Design review of the part built by this model. Coordinates are the model's own, in mm. A direction names the side the tool comes from. Coordinates: 2 decimals unless noted, no trailing zeros. Loops run counter-clockwise (first coordinate to the right, second up) from the corner with the lowest first, then second, coordinate; pieces in that order, holes last. Notation, with made-up numbers: (81, 70.25) -> (102, 70.25) arc R23 ccw to (102, 93.25) -> close; hole circle Ø5 at (57.25, 55.5). An arc over 180 degrees is marked (long way). Use one line per item in the form item = value. Start each with the question number.
1. Wall thickness on line 1 (Y direction, x = 249, z = 26.5); line 2 (Y direction, x = 162, z = -16); line 3 (Z direction, x = 71, y = 4.5): over which ranges is each line inside the solid? List them lowest first. Write a range as from..to.
2. The part is to be moulded in two halves that separate along Y. For faces 5 (the face through (119.259, -30.742, 30.07)), 6 (the face through (120.595, 37.245, 29.93)), 7 (the face through (118, 7, 71)), say which applies: released by +Y, released by -Y, zero draft, split by the parting line, or undercut.
3. For pin 1 (5 mm diameter, centred on x = 209, z = 30, fed in from -Y); pin 2 (6 mm diameter, centred on y = 25.5, z = 31, fed in from +X); pin 3 (5 mm diameter, centred on y = 1.5, z = 3, fed in from +X), all flat-tipped, find the tip position at first contact; note any pin that passes through.
4. Consider section B-B (y = 20.5). State the section outline as (x, z) points, then the cut area to 3 significant figures.
5. Consider section C-C (z = 21.5). State the section outline as (x, y) points, then the cut area to 3 significant figures.
6. Machinability: for faces 1 (the face through (119.281, -29.742, 29.93)), 2 (the face through (251, 7, 31)), 3 (the face through (120, 38, 35)), 4 (the face through (-11, 7, 31)), which of the approach directions +Z, -Z, +X, -X, +Y, -Y give a long, thin tool a straight path to every point of the face, cutting with its end or side? Answer none if there is none.
7. Consider section D-D (y = -3). State the section outline as (x, z) points, then the cut area to 3 significant figures.
8. Consider section A-A (x = 120). State the section outline as (y, z) points, then the cut area to 4 significant figures.
from build123d import *

# Parameters (mm, degrees)
SKETCH1_W           = 262
SKETCH1_H           = 82
BOSS_EXTRUDE1_DEPTH = 10
SKETCH2_W           = 282
SKETCH2_H           = 102
BOSS_EXTRUDE2_DEPTH = 1.25
SKETCH3_R           = 34.5
SKETCH3_R_2         = 33.5
BOSS_EXTRUDE3_DEPTH = 5


with BuildPart() as part:
    # Sketch1 → Boss-Extrude1 (new body)
    with BuildSketch(Plane(origin=(0, 2.5, 0), x_dir=(1, 0, 0), z_dir=(0, 1, 0))):
        with Locations((120, -30)):
            Rectangle(SKETCH1_W, SKETCH1_H)
    extrude(amount=BOSS_EXTRUDE1_DEPTH)

    # Sketch2 → Boss-Extrude2 (add)
    with BuildSketch(Plane(origin=(0, 12.5, 0), x_dir=(1, 0, 0), z_dir=(0, 1, 0))):
        with Locations((120, -30)):
            Rectangle(SKETCH2_W, SKETCH2_H)
    extrude(amount=BOSS_EXTRUDE2_DEPTH)

    # Sketch3 → Boss-Extrude3 (add, symmetric)
    with BuildSketch(Plane.XY.offset(30)):
        with Locations((120, 3.75)):
            Circle(SKETCH3_R)
        with Locations((120, 3.75)):
            Circle(SKETCH3_R_2, mode=Mode.SUBTRACT)
    extrude(amount=BOSS_EXTRUDE3_DEPTH, both=True)


solid = part.part
Geometry check:
q1.line_1 = 2.5..13.75
q1.line_2 = 12.5..13.75
q1.line_3 = -11..71
q2.face_5 = released by -Y
q2.face_6 = undercut
q2.face_7 = zero draft
q3.pin_1 = 2.5
q3.pin_2 = 148.96
q3.pin_3 = 251
q4.outline = (89.84, 25) -> (90.99, 25) -> (90.99, 35) -> (89.84, 35) -> close; (149.01, 25) -> (150.16, 25) -> (150.16, 35) -> (149.01, 35) -> close
q4.area = 23.0 mm²
q5.outline = (-21, 12.5) -> (-11, 12.5) -> (-11, 2.5) -> (251, 2.5) -> (251, 12.5) -> (261, 12.5) -> (261, 13.75) -> (-21, 13.75) -> close
q5.area = 2,970 mm²
q6.face_1 = +Z, -Z
q6.face_2 = +Z, -Z, +X, -Y
q6.face_3 = +Z, +X, -X, +Y
q6.face_4 = +Z, -Z, -X, -Y
q7.outline = (86.17, 25) -> (87.19, 25) -> (87.19, 35) -> (86.17, 35) -> close; (152.81, 25) -> (153.83, 25) -> (153.83, 35) -> (152.81, 35) -> close
q7.area = 20.4 mm²
q8.outline = (-30.75, 25) -> (-29.75, 25) -> (-29.75, 35) -> (-30.75, 35) -> close; (2.5, -11) -> (12.5, -11) -> (12.5, -21) -> (13.75, -21) -> (13.75, 81) -> (12.5, 81) -> (12.5, 71) -> (2.5, 71) -> close; (37.25, 25) -> (38.25, 25) -> (38.25, 35) -> (37.25, 35) -> close
q8.area = 967.5 mm²
